For this review, take the finished solid that the model builds, in its own axes (mm). Give positions to 0.01 mm unless a question says otherwise; leave off trailing zeros. Loops run counter-clockwise (first coordinate to the right, second up) from the corner with the lowest first, then second, coordinate; pieces in that order, holes last.
```python
from build123d import *

# Parameters (mm, degrees)
SKETCH1_W           = 241
SKETCH1_H           = 15
BOSS_EXTRUDE1_DEPTH = 5
SKETCH2_R           = 5
CUT_EXTRUDE2_DEPTH  = 5


with BuildPart() as part:
    # Sketch1 → Boss-Extrude1 (new body)
    with BuildSketch(Plane.XY):
        with Locations((25.298972138, 7.5)):
            Rectangle(SKETCH1_W, SKETCH1_H)
    extrude(amount=BOSS_EXTRUDE1_DEPTH)

    # Sketch2 → Cut-Extrude2 (cut)
    with BuildSketch(Plane.XY.offset(5)):
        with Locations((-87.701027862, 7.5)):
            Circle(SKETCH2_R)
        with BuildLine():
            Line((-87.701027825, 15), (-95.201027862, 15))
            Line((-95.201027862, 15), (-95.201027862, 7.5))
            ThreePointArc((-95.201027862, 7.5), (-93.004328708, 12.803300872), (-87.701027825, 15))
        make_face()
        with BuildLine():
            ThreePointArc((-87.701027862, 0), (-93.004328721, 2.196699141), (-95.201027862, 7.5))
            Line((-95.201027862, 7.5), (-95.201027862, 0))
            Line((-95.201027862, 0), (-87.701027862, 0))
        make_face()
        with Locations((138.298972138, 7.5)):
            Circle(SKETCH2_R)
        with BuildLine():
            Line((145.798972138, 15), (138.298972138, 15))
            ThreePointArc((138.298972138, 15), (143.602272997, 12.803300859), (145.798972138, 7.5))
            Line((145.798972138, 7.5), (145.798972138, 15))
        make_face()
        with BuildLine():
            ThreePointArc((145.798972138, 7.5), (143.602272997, 2.196699141), (138.298972138, 0))
            Line((138.298972138, 0), (145.798972138, 0))
            Line((145.798972138, 0), (145.798972138, 7.5))
        make_face()
    extrude(amount=-CUT_EXTRUDE2_DEPTH, mode=Mode.SUBTRACT)


solid = part.part
```
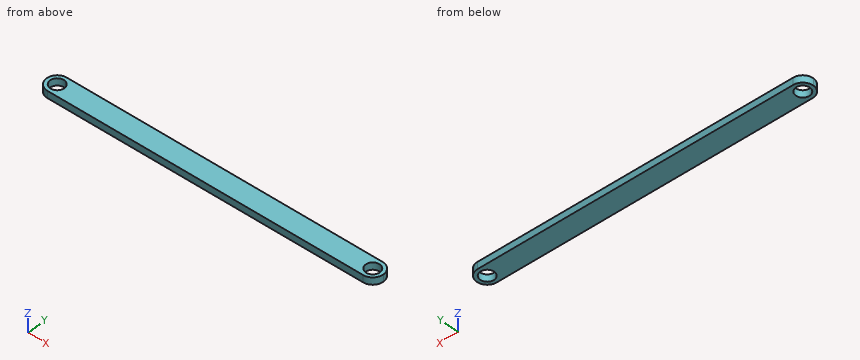
Q1. Consider section A-A on z = 2.45. Give the boundary of the cut face in (x, y).
Answers:
outline: (-87.7, 0) - (138.3, 0) arc R7.5 ccw to (138.3, 15) - (-87.7, 15) arc R7.5 ccw to start; hole circle Ø10 at (-87.7, 7.5); hole circle Ø10 at (138.3, 7.5)
Q2. For pin 1 Ø1.5 at (y, z) = (3.5, 3.5) entering from +X; pin 2 Ø9 at (x, y) = (138.3, 7.5) entering from +Z; pin 3 Ø1 at (y, z) = (5.5, 2.5) entering from -X, all flat-tipped, find the tip position at first contact; note any pin that passes through.
Answers:
pin 1: stops at x = 145.06
pin 2: passes through
pin 3: stops at x = -95.05
Q3. For probe 1 along X at (y, z) = (8.5, 3.3); probe 2 along X at (y, z) = (4.25, 2.25), list the stretches that pass through material, from the lowest coordinate up.
Answers:
probe 1: x = -95.13 to -92.6, -82.8 to 133.4, 143.2 to 145.73
probe 2: x = -94.46 to -91.5, -83.9 to 134.5, 142.1 to 145.06
